Build history of the part. All positions in model axes, mm. Face numbers are marked on the shaded views. A direction names the side the tool comes from. Give positions to 0.01 mm unless a question says otherwise; leave off trailing zeros. Write each loop counter-clockwise with the first axis right and the second up, starting at its lowest first coordinate (ties: lowest second). Pieces come first, ordered by that corner, then holes. Notation, with made-up numbers: (-34, -33.75) -> (-6, -33.75) arc R7 ccw to (-6, -28.75) -> close; hole circle Ø2 at (58.5, 49). An arc over 180 degrees is marked (long way). One line per question, with ' | ' between items. Start each with the question number.
(1) Drill centre lines: probe 1 along X at (y, z) = (-20.75, 31.5); probe 2 along Z at (x, y) = (42.5, -3.25); probe 3 along Z at (x, y) = (39, -18.25). Where is each one in solid material? Low to high. Write a range as from..to.
(2) Band-saw the part on A-A, the plane x = 34.5. Give the cut face in (y, z), and give its area (3 significant figures).
(3) Pull direction Z, two halves, no side cores. Call the marked faces 1, 2 and 3: released by +Z, released by -Z, zero draft, split by the parting line, or undercut.
(4) Band-saw the part on D-D, the plane z = 50. Give the cut face in (x, y).
(5) Band-saw the part on B-B, the plane y = -3. Give the cut face in (x, z).
(6) Tool access for the marked faces 4 and 5: list every direction of +Z, -Z, +X, -X, +Y, -Y with a clear straight run to the whole face (end or side of a thin tool).
(7) Band-saw the part on C-C, the plane z = 10.5. Give the cut face in (x, y), and give its area (3 significant figures).
(8) Pin check, flat tips, straight feed: P1, Ø3, axis at y = -10, z = 42, coming from the +X side; P2, Ø12.5, axis at y = -7.5, z = 19.5, coming from the +X side. Stop position of each tip, or through.
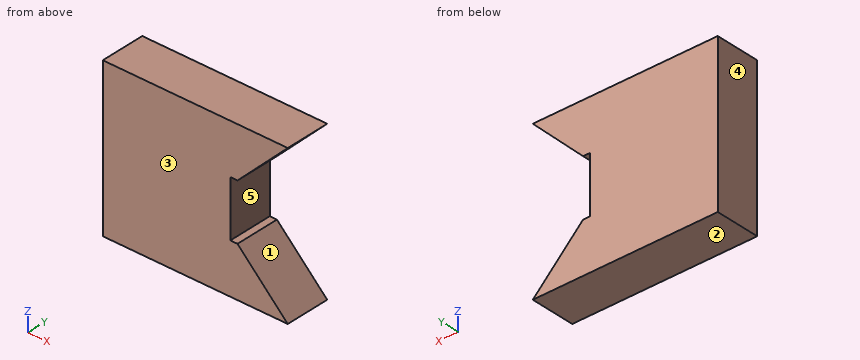
from build123d import *

# Parameters (mm, degrees)
F0_W     = 72.161538
F0_H     = 16.002
F1_DEPTH = 25.4


with BuildPart() as f1:
    # F0 (on Front) → F1 (new body)
    with BuildSketch(Plane.XZ):
        Polygon((-48.940382, 0), (-48.940382, -28.448), (55.707618, -28.448), (27.259618, 0), (23.221156, 0), align=None)
        with Locations((-12.859613, 8.001)):
            Rectangle(F0_W, F0_H)
    extrude(amount=F1_DEPTH)

    # F2: F1 across face


with BuildPart() as f1_1:
    add(f1.part)
    add(f1.part.mirror(Plane(origin=(-12.859613, -12.7, 16.002), x_dir=(1, 0, 0), z_dir=(0, 0, 1))))


solid = f1_1.part
Results:
1) probe 1: x = -48.94..23.22 | probe 2: z = -28.45..-15.24, 47.24..60.45 | probe 3: z = -28.45..-11.74, 43.74..60.45
2) outline: (-25.4, -28.45) -> (0, -28.45) -> (0, -7.24) -> (-25.4, -7.24) -> close; (-25.4, 39.24) -> (0, 39.24) -> (0, 60.45) -> (-25.4, 60.45) -> close | area: 1,080 mm²
3) face 1: undercut | face 2: released by -Z | face 3: zero draft
4) outline: (-48.94, -25.4) -> (45.26, -25.4) -> (45.26, 0) -> (-48.94, 0) -> close
5) outline: (-48.94, -28.45) -> (55.71, -28.45) -> (27.26, 0) -> (23.22, 0) -> (23.22, 32) -> (27.26, 32) -> (55.71, 60.45) -> (-48.94, 60.45) -> close
6) face 4: +Z, -Z, -X, +Y, -Y | face 5: +X, +Y, -Y
7) outline: (-48.94, -25.4) -> (23.22, -25.4) -> (23.22, 0) -> (-48.94, 0) -> close | area: 1,830 mm²
8) P1: stops at x = 38.76 | P2: stops at x = 23.22
